CAD build for the part. Positions are in the model's coordinates, mm. A direction names the side the tool comes from. Give positions to 0.01 mm unless a question says otherwise; leave off trailing zeros. Write each loop counter-clockwise with the first axis right and the second up, starting at its lowest first coordinate (ties: lowest second). Pieces come first, ordered by that corner, then holes. Notation, with made-up numbers: (63.5, 62.25) - (117.5, 62.25) arc R30 ccw to (117.5, 87.25) - close; hole circle Ø7 at (-9, 15). An arc over 180 degrees is marked (long way). Write item = value, one per line. Start each with the question number.
```python
from build123d import *

# Parameters (mm, degrees)
BOSS_EXTRUDE1_DEPTH = 65
SKETCH2_W           = 18
SKETCH2_H           = 76
CUT_EXTRUDE1_DEPTH  = 48.5
CHAMFER1_SIZE       = 10
CHAMFER2_SIZE       = 5
SKETCH3_R           = 15
CUT_EXTRUDE2_DEPTH  = 5
SKETCH5_R           = 1.5
CUT_EXTRUDE3_DEPTH  = 3.75
FILLET1_R           = 1
SKETCH6_W           = 15
SKETCH6_H           = 40
CUT_EXTRUDE4_DEPTH  = 157.644501978
SKETCH7_R           = 1.5
SKETCH7_W           = 15
SKETCH7_H           = 27
CUT_EXTRUDE5_DEPTH  = 10


with BuildPart() as part:
    # Sketch1 → Boss-Extrude1 (new body)
    with BuildSketch(Plane.XY):
        with BuildLine():
            Line((-35, 137.5), (35, 137.5))
            Line((35, 137.5), (37.49377228, 0.68340342))
            ThreePointArc((37.49377228, 0.68340342), (0, -37.5), (-37.49377228, 0.68340342))
            Line((-37.49377228, 0.68340342), (-35, 137.5))
        make_face()
    extrude(amount=BOSS_EXTRUDE1_DEPTH)

    # Sketch2 → Cut-Extrude1 (cut, symmetric)
    with BuildSketch(Plane(origin=(0, 0, 0), x_dir=(0, 0, -1), z_dir=(1, 0, 0))):
        with Locations((-56, 0.5)):
            Rectangle(SKETCH2_W, SKETCH2_H)
        with Locations((-9, 0.5)):
            Rectangle(SKETCH2_W, SKETCH2_H)
    extrude(amount=CUT_EXTRUDE1_DEPTH, both=True, mode=Mode.SUBTRACT)

    # Chamfer1
    chamfer1_edges = [part.edges().sort_by_distance(p)[0] for p in [
        (-35.902242352, 88, 65),
        (35.902242352, 88, 0),
        (35.902242352, 88, 65),
        (-35.902242352, 88, 0),
    ]]
    chamfer(chamfer1_edges, length=CHAMFER1_SIZE)

    # Chamfer2
    chamfer2_edges = [part.edges().sort_by_distance(p)[0] for p in [
        (0, -37.5, 18),
        (0, -37.5, 47),
        (37.149128492, 19.59170171, 47),
        (-37.149128492, 19.59170171, 47),
        (37.149128492, 19.59170171, 18),
        (-37.149128492, 19.59170171, 18),
    ]]
    chamfer(chamfer2_edges, length=CHAMFER2_SIZE)

    # Sketch3 → Cut-Extrude2 (cut, symmetric)
    with BuildSketch(Plane.XY.offset(47)):
        Circle(SKETCH3_R)
    extrude(amount=CUT_EXTRUDE2_DEPTH, both=True, mode=Mode.SUBTRACT)

    # Sketch5 → Cut-Extrude3 (cut, symmetric)
    with BuildSketch(Plane.XY.offset(42)):
        with Locations((0, 7.5)):
            Circle(SKETCH5_R)
        with Locations((7.5, 0)):
            Circle(SKETCH5_R)
        with Locations((0, -7.5)):
            Circle(SKETCH5_R)
        with Locations((-7.5, 0)):
            Circle(SKETCH5_R)
    extrude(amount=CUT_EXTRUDE3_DEPTH, both=True, mode=Mode.SUBTRACT)

    # Fillet1
    fillet1_edges = [part.edges().sort_by_distance(p)[0] for p in [
        (-15, 0, 47),
        (-15, 0, 42),
    ]]
    fillet(fillet1_edges, radius=FILLET1_R)

    # Sketch6 → Cut-Extrude4 (cut, through all)
    with BuildSketch(Plane.XY.offset(65)):
        with Locations((0, 107.5)):
            Rectangle(SKETCH6_W, SKETCH6_H)
    extrude(amount=-CUT_EXTRUDE4_DEPTH, mode=Mode.SUBTRACT)

    # Sketch7 → Cut-Extrude5 (cut)
    with BuildSketch(Plane(origin=(0, 137.5, 0), x_dir=(1, 0, 0), z_dir=(0, 1, 0))):
        with Locations(Location((-3.25, -15.75, 0), (0, 0, 270))):
            Circle(SKETCH7_R)
        with Locations(Location((3.25, -15.75, 0), (0, 0, 270))):
            Circle(SKETCH7_R)
        with Locations(Location((3.25, -49.25, 0), (0, 0, 270))):
            Circle(SKETCH7_R)
        with Locations(Location((-3.25, -49.25, 0), (0, 0, 270))):
            Circle(SKETCH7_R)
        with Locations((0, -32.5)):
            Rectangle(SKETCH7_W, SKETCH7_H)
    extrude(amount=-CUT_EXTRUDE5_DEPTH, mode=Mode.SUBTRACT)


solid = part.part
```
1. Cut at B-B (y = 22). Give the cut face in (x, z), then the cut area to 3 significant figures.
2. Tool access for faces 4 (the flat face through (0, 87.5, 33)), 5 (the cylindrical face through (-14.985, 0.66, 44.521)), 6 (the flat face through (0, 18, 47)), 7 (the flat face through (0, 133, 19)), 8 (the flat face through (0, 3, 18)): list every direction of +Z, -Z, +X, -X, +Y, -Y with a clear straight run to the whole face (end or side of a thin tool).
3. Pin check, flat tips, straight feed: pin 1 Ø12 at (y, z) = (100.5, 57.5) entering from -X; pin 2 Ø12 at (x, z) = (24.5, 22) entering from -Y; pin 3 Ø4.5 at (x, z) = (-2, 59) entering from -Y. Stop position of each tip, or through.
4. Wall check: line 1 along X through (y, z) = (134, 15.75); line 2 along Z through (x, y) = (18.5, 6.5); line 3 along Z through (x, y) = (2, -10.5). Give the ranges that are in metal, low to high.
5. Cut at A-A (y = 47). Give the cut face in (x, z).
6. Mould opens along Y. For faces 1 (the flat face through (0, 78, 65)), 2 (the flat face through (-8, 137.5, 32)), 3 (the flat face through (0, 127.5, 10)) say: +Y half, -Y half, draft (parallel to the pull), parting line (faces both ways), or undercut.
Output:
q1.outline = (-37.11, 23) - (-32.1, 18) - (32.1, 18) - (37.11, 23) - (37.11, 42) - (32.1, 47) - (-32.1, 47) - (-37.11, 42) - close
q1.area = 2,100 mm2
q2.face_4 = +Z, -Z
q2.face_5 = +Z
q2.face_6 = +Z, +X, -X, -Y
q2.face_7 = +Y
q2.face_8 = -Z, +X, -X, -Y
q3.pin_1 = -35.77
q3.pin_2 = -32.57
q3.pin_3 = 38.5
q4.line_1 = -35.06 to -4.75, -1.75 to 1.75, 4.75 to 35.06
q4.line_2 = 18 to 47
q4.line_3 = 18 to 42
q5.outline = (-36.65, 10) - (-26.65, 0) - (26.65, 0) - (36.65, 10) - (36.65, 55) - (26.65, 65) - (-26.65, 65) - (-36.65, 55) - close
q6.face_1 = draft
q6.face_2 = +Y half
q6.face_3 = undercut
